from build123d import *

# Parameters (mm, degrees)
F0_W     = 49.1559793526
F0_H     = 6.35
F0_W_2   = 5.08
F0_W_3   = 23.8690206474
F1_DEPTH = 1.27
F2_DEPTH = 25.4
F3_W     = 5.08
F3_H     = 12.7
F4_DEPTH = 42.624
F6_DEPTH = 25.4
F7_R     = 3.175
F8_DEPTH = 25.4


with BuildPart() as f1:
    # F0 (on Top) → F1 (new body)
    with BuildSketch(Plane.XY):
        with Locations((-50.9870103237, -50.419)):
            Rectangle(F0_W, F0_H)
        Polygon((-75.565, 47.244), (-2.54, 47.244), (-2.54, 53.594), (-81.915, 53.594), (-81.915, -53.594), (-75.565, -53.594), (-75.565, -47.244), align=None)
        with Locations((0, 56.769)):
            Rectangle(F0_W_2, F0_H)
        with Locations((0, 50.419)):
            Rectangle(F0_W_2, F0_H)
        Polygon((2.54, 47.244), (75.565, 47.244), (75.565, -47.244), (75.565, -53.594), (81.915, -53.594), (81.915, 53.594), (2.54, 53.594), align=None)
        with Locations((50.9870103237, -50.419)):
            Rectangle(F0_W, F0_H)
        with Locations((-14.4745103237, -50.419)):
            Rectangle(F0_W_3, F0_H)
        with Locations((0, -50.419)):
            Rectangle(F0_W_2, F0_H)
        with Locations((14.4745103237, -50.419)):
            Rectangle(F0_W_3, F0_H)
        with Locations((0, -56.769)):
            Rectangle(F0_W_2, F0_H)
    extrude(amount=F1_DEPTH)

    # F0 (on Top) → F2 (join)
    with BuildSketch(Plane.XY):
        Polygon((-75.565, 47.244), (-2.54, 47.244), (-2.54, 53.594), (-81.915, 53.594), (-81.915, -53.594), (-75.565, -53.594), (-75.565, -47.244), align=None)
        with Locations((0, 56.769)):
            Rectangle(F0_W_2, F0_H)
        with Locations((0, 50.419)):
            Rectangle(F0_W_2, F0_H)
        Polygon((2.54, 47.244), (75.565, 47.244), (75.565, -47.244), (75.565, -53.594), (81.915, -53.594), (81.915, 53.594), (2.54, 53.594), align=None)
        with Locations((14.4745103237, -50.419)):
            Rectangle(F0_W_3, F0_H)
        with Locations((0, -50.419)):
            Rectangle(F0_W_2, F0_H)
        with Locations((-14.4745103237, -50.419)):
            Rectangle(F0_W_3, F0_H)
        with Locations((0, -56.769)):
            Rectangle(F0_W_2, F0_H)
    extrude(amount=F2_DEPTH)

    # F3 (on face) → F4 (join)
    with BuildSketch(Plane.XY.offset(25.4)):
        Polygon((2.54, 59.944), (-2.54, 59.944), (-2.54, 53.594), (-2.54, 47.244), (2.54, 47.244), (2.54, 53.594), align=None)
        with Locations((0, -53.594)):
            Rectangle(F3_W, F3_H)
    extrude(amount=F4_DEPTH)

    # F5 (on face) → F6 (cut)
    with BuildSketch(Plane.YZ.offset(2.54)):
        with BuildLine():
            Line((-58.2624942683, 8.2038091254), (-58.2624942683, 8.1145596807))
            ThreePointArc((-58.2624942683, 8.1145596807), (-56.7408433733, 6.6593503961), (-55.2631582039, 8.159184403))
            ThreePointArc((-55.2631582039, 8.159184403), (-55.4440615048, 8.8733159724), (-55.9431367352, 9.4151958643))
            ThreePointArc((-55.9431367352, 9.4151958643), (-56.7631582039, 9.1712073255), (-57.5831796726, 9.4151958643))
            ThreePointArc((-57.5831796726, 9.4151958643), (-58.0714851124, 8.8928605581), (-58.2624942683, 8.2038091254))
        make_face()
        with BuildLine():
            ThreePointArc((-58.2624942683, 8.2038091254), (-58.2631582039, 8.159184403), (-58.2624942683, 8.1145596807))
            Line((-58.2624942683, 8.1145596807), (-58.2624942683, 8.2038091254))
        make_face()
        with BuildLine():
            ThreePointArc((-55.9431367352, 9.4151958643), (-55.4440615048, 8.8733159724), (-55.2631582039, 8.159184403))
            Line((-55.2631582039, 8.159184403), (-55.2631582039, 10.6712073255))
            ThreePointArc((-55.2631582039, 10.6712073255), (-55.4440615048, 9.9570757561), (-55.9431367352, 9.4151958643))
        make_face()
        with BuildLine():
            Line((-58.2624942683, 10.6265826032), (-58.2624942683, 8.2038091254))
            ThreePointArc((-58.2624942683, 8.2038091254), (-58.0714851124, 8.8928605581), (-57.5831796726, 9.4151958643))
            ThreePointArc((-57.5831796726, 9.4151958643), (-58.0714851124, 9.9375311705), (-58.2624942683, 10.6265826032))
        make_face()
        with BuildLine():
            ThreePointArc((-57.5831796726, 9.4151958643), (-56.7631582039, 9.659184403), (-55.9431367352, 9.4151958643))
            ThreePointArc((-55.9431367352, 9.4151958643), (-55.4440615048, 9.9570757561), (-55.2631582039, 10.6712073255))
            ThreePointArc((-55.2631582039, 10.6712073255), (-56.7854730345, 12.1710413325), (-58.2624942683, 10.6265826032))
            ThreePointArc((-58.2624942683, 10.6265826032), (-58.0714851124, 9.9375311705), (-57.5831796726, 9.4151958643))
        make_face()
        with BuildLine():
            ThreePointArc((-57.5831796726, 9.4151958643), (-56.7631582039, 9.1712073255), (-55.9431367352, 9.4151958643))
            ThreePointArc((-55.9431367352, 9.4151958643), (-56.7631582039, 9.659184403), (-57.5831796726, 9.4151958643))
        make_face()
    extrude(amount=-F6_DEPTH, mode=Mode.SUBTRACT)

    # F7 (on face) → F8 (cut)
    with BuildSketch(Plane.YZ.offset(2.54)):
        with Locations((53.594, 58.674)):
            Circle(F7_R)
        with BuildLine():
            ThreePointArc((-50.419, 58.674), (-52.3789801022, 61.6073175157), (-55.8390640303, 60.9190640303))
            Line((-55.8390640303, 60.9190640303), (-51.3489359697, 56.4289359697))
            ThreePointArc((-51.3489359697, 56.4289359697), (-50.6606824843, 57.4589801022), (-50.419, 58.674))
        make_face()
        with BuildLine():
            Line((-51.3489359697, 56.4289359697), (-55.8390640303, 60.9190640303))
            ThreePointArc((-55.8390640303, 60.9190640303), (-55.8390640303, 56.4289359697), (-51.3489359697, 56.4289359697))
        make_face()
    extrude(amount=-F8_DEPTH, mode=Mode.SUBTRACT)


solid = f1.part
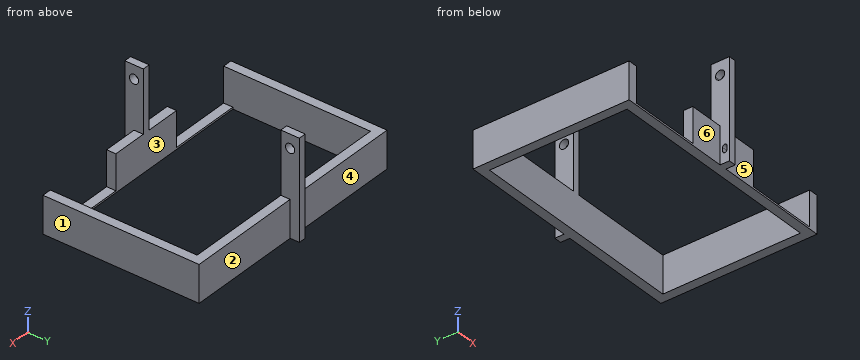
CAD build for the part. Positions are in the model's coordinates, mm. Face numbers are marked on the shaded views. A direction names the side the tool comes from. Give positions to 0.01 mm unless a question says otherwise; leave off trailing zeros. Write each loop counter-clockwise with the first axis right and the second up, starting at its lowest first coordinate (ties: lowest second). Pieces come first, ordered by that corner, then holes. Notation, with made-up numbers: M 83.5,4 L 128.5,4 A26 cw 128.5,27 Z; hole C -30.75,71 d6. An arc over 180 degrees is marked long. Put each result on its own line as item: value. Start each with the question number.
(1) Band-saw the part on B-B, the plane y = 34. Write the cut outline in (x, z) (3 decimals).
(2) Band-saw the part on A-A, the plane x = 6. Write the cut outline in (y, z).
(3) Mould opens along Y. For the marked faces 1, 2 and 3 say: +Y half, -Y half, draft (parallel to the pull), parting line (faces both ways), or undercut.
(4) Band-saw the part on C-C, the plane z = 15.5. Write the cut outline in (x, y) (3 decimals).
(5) Probe L1, parallel to Z at x = 1, y = -53.5; L2, parallel to Y at x = 25, z = 8; L3, parallel to Y at x = 55, z = 13. List the from-to ranges inside material, lowest first.
(6) Flat gauge pins, fed straight in: pin 1 Ø10 at (y, z) = (54, 37) entering from +X; pin 2 Ø12.5 at (x, z) = (-40.5, 7) entering from -Y; pin 3 Ø4 at (x, z) = (44, 19) entering from -Y. Where does each tip first touch, or does it go through?
(7) Which spindle directions (+Z, -Z, +X, -X, +Y, -Y) get a long thin tool onto all of the face, cutting with end or side? Do the marked faces 4, 5 and 6. Say none if no direction does.
Response values:
1. outline: M -81.915,0 L -75.565,0 L -75.565,25.4 L -81.915,25.4 Z; M 75.565,0 L 81.915,0 L 81.915,25.4 L 75.565,25.4 Z
2. outline: M -53.59,0 L -47.24,0 L -47.24,25.4 L -53.59,25.4 Z; M 47.24,0 L 53.59,0 L 53.59,25.4 L 47.24,25.4 Z
3. face 1: draft
3. face 2: +Y half
3. face 3: undercut
4. outline: M -81.915,-53.594 L -75.565,-53.594 L -75.565,47.244 L 75.565,47.244 L 75.565,-53.594 L 81.915,-53.594 L 81.915,53.594 L 2.54,53.594 L 2.54,59.944 L -2.54,59.944 L -2.54,53.594 L -81.915,53.594 Z; M -26.409,-53.594 L -2.54,-53.594 L -2.54,-59.944 L 2.54,-59.944 L 2.54,-53.594 L 26.409,-53.594 L 26.409,-47.244 L -26.409,-47.244 Z
5. L1: z = 0 to 55.5, 61.85 to 68.02
5. L2: y = -53.59 to -47.24, 47.24 to 53.59
5. L3: y = 47.24 to 53.59
6. pin 1: stops at x = 2.54
6. pin 2: stops at y = -53.59
6. pin 3: stops at y = 47.24
7. face 4: +Z, -Z, -X, +Y
7. face 5: +Z, -Z, +X, -Y
7. face 6: +Z, -Z, -X, -Y
